Autodesk Inventor part; units mm, degrees
ref_plane "YZ Plane" through (0, 0, 0) normal (1, 0, 0) x (0, 1, 0)
ref_plane "XZ Plane" through (0, 0, 0) normal (0, 1, 0) x (-1, 0, 0)
ref_plane "XY Plane" through (0, 0, 0) normal (0, 0, 1) x (1, 0, 0)
sketch "Sketch1" plane through (0, 0, 0) normal (0, 1, 0) x (-1, 0, 0)
  arc A0 (39.6019, 0) -> (55.3297, -52.2069) centre (134.1138, 0) ccw
  circle A1 centre (28.625, -37.55) radius 1.75
  circle A2 centre (25.375, -42.175) radius 1.75
  circle A3 centre (46.65, -60.8866) radius 4.25
  arc A4 (37.9702, -69.5664) -> (55.3297, -52.2069) centre (46.65, -60.8866) ccw
  arc A5 (37.9702, -69.5664) -> (0, -53.8386) centre (0, -107.5366) ccw
  line L0 (28.315, -9.4519) -> (0.0544, -9.4519)
  arc A6 (28.315, -9.4519) -> (28.625, -9.4382) centre (28.315, -5.9519) ccw
  arc A7 (28.315, -9.4519) -> (31.815, -5.9519) centre (28.315, -5.9519) ccw
  line L1 (31.815, 0) -> (31.815, -5.9519)
  circle A8 centre (46.65, -60.8866) radius 4.25
  circle A9 centre (25.375, -42.175) radius 1.75
  circle A10 centre (28.625, -37.55) radius 1.75
  arc A11 (39.6019, 0) -> (55.3297, -52.2069) centre (134.1138, 0) ccw
  arc A12 (37.9702, -69.5664) -> (0, -53.8386) centre (0, -107.5366) ccw
  line L2 (39.6019, 0) -> (0, 0) construction
  line L3 (0, -18.3592) -> (21.875, -18.3592)
  line L4 (25.375, -21.8592) -> (25.375, -24.8427)
  line L5 (21.875, -28.3427) -> (0, -28.3427)
  arc A13 (25.375, -21.8592) -> (21.875, -18.3592) centre (21.875, -21.8592) ccw
  arc A14 (21.875, -28.3427) -> (25.375, -24.8427) centre (21.875, -24.8427) ccw
  arc A15 (0, -42.175) -> (0, -38.675) centre (0, -40.425) ccw
  line L6 (0, -53.8386) -> (0, -42.175) construction
  line L7 (31.815, 0) -> (31.815, 5.9519)
  arc A16 (31.815, 5.9519) -> (28.315, 9.4519) centre (28.315, 5.9519) ccw
  arc A17 (28.625, 9.4382) -> (28.315, 9.4519) centre (28.315, 5.9519) ccw
  line L8 (28.315, 9.4519) -> (0.0544, 9.4519)
  arc A18 (55.3297, 52.2069) -> (39.6019, 0) centre (134.1138, 0) ccw
  circle A19 centre (28.625, 37.55) radius 1.75
  circle A20 centre (25.375, 42.175) radius 1.75
  arc A21 (0, 53.8386) -> (37.9702, 69.5664) centre (0, 107.5366) ccw
  circle A22 centre (46.65, 60.8866) radius 4.25
  arc A23 (55.3297, 52.2069) -> (37.9702, 69.5664) centre (46.65, 60.8866) ccw
  circle A24 centre (46.65, 60.8866) radius 4.25
  circle A25 centre (25.375, 42.175) radius 1.75
  circle A26 centre (28.625, 37.55) radius 1.75
  arc A27 (55.3297, 52.2069) -> (39.6019, 0) centre (134.1138, 0) ccw
  arc A28 (0, 53.8386) -> (37.9702, 69.5664) centre (0, 107.5366) ccw
  line L9 (0, 18.3592) -> (21.875, 18.3592)
  line L10 (25.375, 21.8592) -> (25.375, 24.8427)
  line L11 (21.875, 28.3427) -> (0, 28.3427)
  arc A29 (21.875, 18.3592) -> (25.375, 21.8592) centre (21.875, 21.8592) ccw
  arc A30 (25.375, 24.8427) -> (21.875, 28.3427) centre (21.875, 24.8427) ccw
  arc A31 (0, 38.675) -> (0, 42.175) centre (0, 40.425) ccw
  line L12 (0, 53.8386) -> (0, 42.175) construction
  line L13 (0, 38.675) -> (0, 0) construction
  line L14 (-31.815, 0) -> (-31.815, -5.9519)
  arc A32 (-31.815, -5.9519) -> (-28.315, -9.4519) centre (-28.315, -5.9519) ccw
  arc A33 (-28.625, -9.4382) -> (-28.315, -9.4519) centre (-28.315, -5.9519) ccw
  line L15 (-28.315, -9.4519) -> (-0.0544, -9.4519)
  arc A34 (-55.3297, -52.2069) -> (-39.6019, 0) centre (-134.1138, 0) ccw
  circle A35 centre (-28.625, -37.55) radius 1.75
  circle A36 centre (-25.375, -42.175) radius 1.75
  arc A37 (0, -53.8386) -> (-37.9702, -69.5664) centre (0, -107.5366) ccw
  circle A38 centre (-46.65, -60.8866) radius 4.25
  arc A39 (-55.3297, -52.2069) -> (-37.9702, -69.5664) centre (-46.65, -60.8866) ccw
  circle A40 centre (-46.65, -60.8866) radius 4.25
  circle A41 centre (-25.375, -42.175) radius 1.75
  circle A42 centre (-28.625, -37.55) radius 1.75
  arc A43 (-55.3297, -52.2069) -> (-39.6019, 0) centre (-134.1138, 0) ccw
  arc A44 (0, -53.8386) -> (-37.9702, -69.5664) centre (0, -107.5366) ccw
  line L16 (0, -18.3592) -> (-21.875, -18.3592)
  line L17 (-25.375, -21.8592) -> (-25.375, -24.8427)
  line L18 (-21.875, -28.3427) -> (0, -28.3427)
  arc A45 (-21.875, -18.3592) -> (-25.375, -21.8592) centre (-21.875, -21.8592) ccw
  arc A46 (-25.375, -24.8427) -> (-21.875, -28.3427) centre (-21.875, -24.8427) ccw
  arc A47 (0, -38.675) -> (0, -42.175) centre (0, -40.425) ccw
  line L19 (0, 18.3592) -> (-21.875, 18.3592)
  arc A48 (-25.375, 21.8592) -> (-21.875, 18.3592) centre (-21.875, 21.8592) ccw
  line L20 (-28.315, 9.4382) -> (-0.0544, 9.445)
  arc A49 (-28.315, 9.4382) -> (-31.815, 5.9519) centre (-28.315, 5.9382) ccw
  line L21 (-31.815, 0) -> (-31.815, 5.9519)
  arc A50 (-28.315, 9.4382) -> (-28.6259, 9.4244) centre (-28.315, 5.9382) ccw
  arc A51 (-37.9702, 69.5664) -> (0, 53.8386) centre (0, 107.5366) ccw
  arc A52 (-37.9702, 69.5664) -> (0, 53.8386) centre (0, 107.5366) ccw
  circle A53 centre (-46.65, 60.8866) radius 4.25
  circle A54 centre (-46.65, 60.8866) radius 4.25
  arc A55 (-37.9702, 69.5664) -> (-55.3297, 52.2069) centre (-46.65, 60.8866) ccw
  arc A56 (-21.875, 28.3427) -> (-25.375, 24.8427) centre (-21.875, 24.8427) ccw
  circle A57 centre (-28.625, 37.55) radius 1.75
  circle A58 centre (-25.375, 42.175) radius 1.75
  circle A59 centre (-25.375, 42.175) radius 1.75
  line L22 (-21.875, 28.3427) -> (0, 28.3427)
  arc A60 (0, 42.175) -> (0, 38.675) centre (0, 40.425) ccw
  arc A61 (-39.6019, 0) -> (-55.3297, 52.2069) centre (-134.1138, 0) ccw
  circle A62 centre (-28.625, 37.55) radius 1.75
  line L23 (-25.375, 21.8592) -> (-25.375, 24.8427)
  arc A63 (-39.6019, 0) -> (-55.3297, 52.2069) centre (-134.1138, 0) ccw
  circle A64 centre (-25.5, 34.24) radius 1.75
  circle A65 centre (-25.5, -34.24) radius 1.75
  circle A66 centre (25.5, 34.24) radius 1.75
  circle A67 centre (25.5, -34.24) radius 1.75
  arc A68 (-37.9702, 69.5664) -> (-55.3297, 52.2069) centre (-46.65, 60.8866) ccw
  arc A69 (-55.3297, -52.2069) -> (-37.9702, -69.5664) centre (-46.65, -60.8866) ccw
  arc A70 (55.3297, 52.2069) -> (37.9702, 69.5664) centre (46.65, 60.8866) ccw
  arc A71 (37.9702, -69.5664) -> (55.3297, -52.2069) centre (46.65, -60.8866) ccw
  arc A72 (-37.9702, 69.5664) -> (37.9702, 69.5664) centre (0, 107.5366) ccw
  arc A73 (37.9702, -69.5664) -> (-37.9702, -69.5664) centre (0, -107.5366) ccw
  arc A74 (-55.3297, -52.2069) -> (-55.3297, 52.2069) centre (-134.1138, 0) ccw
  arc A75 (55.3297, 52.2069) -> (55.3297, -52.2069) centre (134.1138, 0) ccw
  line L24 (-21.875, 28.3427) -> (21.875, 28.3427)
  line L25 (21.875, 18.3592) -> (-21.875, 18.3592)
  line L26 (-25.375, 24.8427) -> (-25.375, 21.8592)
  line L27 (25.375, 24.8427) -> (25.375, 21.8592)
  line L28 (-28.315, 9.4382) -> (28.625, 9.4382)
  line L29 (28.625, -9.4382) -> (-28.625, -9.4382)
  line L30 (-31.815, 5.9519) -> (-31.815, -5.9519)
  line L31 (31.815, 5.9519) -> (31.815, -5.9519)
  line L32 (-21.875, -18.3592) -> (21.875, -18.3592)
  line L33 (21.875, -28.3427) -> (-21.875, -28.3427)
  line L34 (-25.375, -21.8592) -> (-25.375, -24.8427)
  line L35 (25.375, -21.8592) -> (25.375, -24.8427)
  arc A76 (-21.875, 28.3427) -> (-25.375, 24.8427) centre (-21.875, 24.8427) ccw
  arc A77 (-25.375, 21.8592) -> (-21.875, 18.3592) centre (-21.875, 21.8592) ccw
  arc A78 (25.375, 24.8427) -> (21.875, 28.3427) centre (21.875, 24.8427) ccw
  arc A79 (21.875, 18.3592) -> (25.375, 21.8592) centre (21.875, 21.8592) ccw
  circle A80 centre (0, 40.425) radius 1.75
  circle A81 centre (0, -40.425) radius 1.75
  point P0 (55.3297, 52.2069)
  point P1 (25.25, -18.3592)
  point P2 (4.2075, -54.5249)
  point P3 (-37.9702, -69.5664)
  point P4 (25.25, 18.3592)
  point P5 (4.2075, 54.5249)
  point P6 (-25.25, -18.3592)
  point P7 (-4.2075, -54.5249)
  point P8 (-25.25, 18.3592)
  point P9 (-4.2075, 54.5249)
  dimension "d93" = 3.5
  dimension "d94" = 37.55
  dimension "d95" = 4.625
  dimension "d96" = 3.5
  dimension "d97" = 3.5
  dimension "d98" = 8.5
  dimension "d100" = 3.5
  dimension "d105" = 3.5
  dimension "d106" = 3.5
  dimension "d107" = 3.5
  dimension "d108" = 3.5
extrude "Extrusion7" add sketch "Sketch1" along normal blind 3.5
sketch "Sketch8" plane through (0, 0, 0) normal (0, -1, 0) x (1, 0, 0)
  circle A0 centre (35.7085, -13.8987) radius 1.75
  circle A1 centre (-35.7085, -13.8987) radius 1.75
  circle A2 centre (35.7085, 13.8987) radius 1.75
  circle A3 centre (-35.7085, 13.8987) radius 1.75
  circle A4 centre (46.65, -60.8866) radius 4.25
  dimension "d120" = 46.9879
  dimension "d121" = 10.9415
extrude "Extrusion8" cut sketch "Sketch8" against normal through all contours A0 | A1 | A2 | A3
properties part number "BAWAH4"
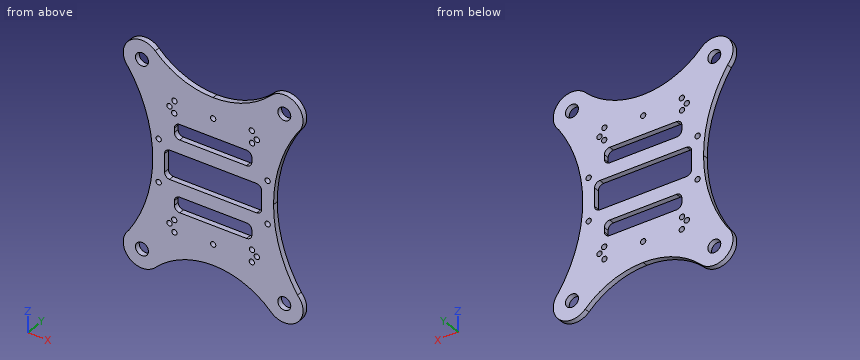
Verification items for the finished model (mm, model axes). Round coordinates to 2 decimals unless told otherwise and drop trailing zeros. Write each loop counter-clockwise with the first axis right and the second up, starting at its lowest first coordinate (ties: lowest second). Pieces come first, ordered by that corner, then holes.
1. Section check C-C on y = 2.9. State how many separate pieces and enclosed holes the cut face has, plus the area to 3 significant figures.
2. Section check B-B on x = 46.65. Enter the section's corners in (y, z), plus the area to 3 significant figures.
3. Scan lines: L1, parallel to Z at x = -46.65, y = 1.7; L2, parallel to Z at x = 0, y = 0.9 (3 decimals); L3, parallel to Z at x = -50, y = 1.5. Record each from-to range of solid material in increasing order.
4. Section check A-A on z = -34.24. Enter the section's corners in (x, y), plus the area to 3 significant figures.
5. Gauge pin test, flat ends, axial feed: P1, Ø1, axis at x = 20.5, y = 1, coming from the -Z side; P2, Ø4, axis at x = 28.625, z = -37.55, coming from the -Y side; P3, Ø1.5, axis at y = 1.5, z = 24, coming from the +X side; P4, Ø0.9, axis at y = 1.5, z = 23.5, coming from the -X side. Record the tip position at first contact, or that the pin passes through.
Answer:
1. separate pieces: 1
1. enclosed holes: 25
1. area: 9,280 mm2
2. outline: (0, -73.16) - (3.5, -73.16) - (3.5, -65.14) - (0, -65.14) - close; (0, -56.64) - (3.5, -56.64) - (3.5, -35.81) - (0, -35.81) - close; (0, 35.81) - (3.5, 35.81) - (3.5, 56.64) - (0, 56.64) - close; (0, 65.14) - (3.5, 65.14) - (3.5, 73.16) - (0, 73.16) - close
2. area: 202 mm2
3. L1: z = -73.16 to -65.14, -56.64 to -35.81, 35.81 to 56.64, 65.14 to 73.16
3. L2: z = -53.839 to -42.175, -38.675 to -28.343, -18.359 to -9.438, 9.438 to 18.359, 28.343 to 38.675, 42.175 to 53.839
3. L3: z = -72.7 to -63.5, -58.27 to -43.1, 43.1 to 58.27, 63.5 to 72.7
4. outline: (-46.02, 0) - (-27.25, 0) - (-27.25, 3.5) - (-46.02, 3.5) - close; (-23.75, 0) - (23.75, 0) - (23.75, 3.5) - (-23.75, 3.5) - close; (27.25, 0) - (46.02, 0) - (46.02, 3.5) - (27.25, 3.5) - close
4. area: 298 mm2
5. P1: stops at z = -58.12
5. P2: stops at y = 0
5. P3: stops at x = 42.9
5. P4: stops at x = -42.69
